The model under review builds one solid part; all positions refer to its coordinate system, in mm. A direction names the side the tool comes from. Round coordinates to 2 decimals unless told otherwise and drop trailing zeros. Order: outer loops, then holes, each group sorted by start corner. A loop starts at its lowest first (then second) coordinate and runs counter-clockwise, first axis right, second up. Notation, with made-up numbers: (60, -35) -> (109, -35) arc R23 ccw to (109, -22) -> close; hole circle Ø8 at (-17, 61.5). An arc over 180 degrees is marked (long way). Use a Markdown table: item, result. Add a question column.
```python
from build123d import *

# Parameters (mm, degrees)
F1_DEPTH = 25.4
F2_DEPTH = 25.4


with BuildPart() as f1:
    # F0 (on Front) → F1 (new body)
    with BuildSketch(Plane.XZ):
        Polygon((-174.676194787, -63.6054873466), (-136.6764605045, -58.7648972869), (-154.4505208731, -22.218702361), (-142.8054571152, 37.529643625), (-136.6764605045, 37.9512919024), (-124.7218182419, 38.7737192321), (60.676984489, 51.5283495188), (90.0961384177, 81.2006369233), (-136.6764605045, 63.0854219198), (-164.5756051188, 29.4337924282), align=None)
        Polygon((-124.7218182419, 38.7737192321), (-136.6764605045, 37.9512919024), (-66.8059885502, -58.7648972869), (-56.2220695239, -45.9986950765), align=None)
        Polygon((90.0961384177, 63.0854219198), (90.0961384177, 81.2006369233), (60.676984489, 51.5283495188), (62.1969938034, 29.4337924282), align=None)
    extrude(amount=F1_DEPTH)

    # F2 (add): a face of the model
    f2_faces = [f1.faces().sort_by_distance(p)[0] for p in [
        (-166.6256944507, -25.4, -17.4115576837),
    ]]
    extrude(f2_faces, amount=F2_DEPTH)


solid = f1.part
```
Q1. Wall thickness on line 1 (X direction, y = -38, z = -10); line 2 (Z direction, x = -74, y = -15.5); line 3 (X direction, y = -17.5, z = -11.5): over which ranges is each line inside the solid? List them lowest first. Write a range as [from, to].
Q2. Add section D-D (x = 11.5). Write out the cut boundary in (y, z), then the cut area to 3 significant figures.
Q3. Add section A-A (x = -146). Write out the cut boundary in (y, z).
Q4. Mouldability with a two-part tool opening along Z and no side actions: class faces 1 (the flat face through (-61.588, -25.044, -52.471)), 2 (the flat face through (90.096, -25, 72)), 3 (the flat face through (-148.71, -25.04, 7.24)) as pulls with the +Z half, pulls with the -Z half, needs draft (parallel to the pull), parting line crosses it, or undercut.
Q5. Add section C-C (z = 47). Write out the cut boundary in (x, y).
Q6. Add section B-B (y = -15.5). Write out the cut boundary in (x, z), then the cut area to 3 significant figures.
Q7. Insertion check: pin 1 (10 mm diameter, centred on x = -0.5, y = -44, fed in from -Z); pin 2 (1 mm diameter, centred on y = -12, z = -4.5, fed in from -X); pin 3 (1.5 mm diameter, centred on x = 10.5, y = -34, fed in from +Z). Each pin has a flat end and moves straight along its axis. Give the tip position at first contact, or say it passes through.
Q8. Machinability: for faces 4 (the flat face through (75.95, -25.04, 46.02)), 5 (the flat face through (61.426, -25.044, 40.636)), 6 (the flat face through (-139.784, -25.044, 37.738)), which of the approach directions +Z, -Z, +X, -X, +Y, -Y give a long, thin tool a straight path to every point of the face, cutting with its end or side? Answer none if there is none.
Report:
| question | item | result |
|---|---|---|
| 1 | line 1 | x = [-168.86, -152.07], [-102.04, -85.31] |
| 1 | line 2 | z = [-48.81, -24], [42.26, 68.09] |
| 1 | line 3 | x = [-169.02, -152.36], [-100.95, -84.1] |
| 2 | outline | (-50.8, 48.15) -> (0, 48.15) -> (0, 74.92) -> (-50.8, 74.92) -> close |
| 2 | area | 1,360 mm² |
| 3 | outline | (-50.8, -59.95) -> (0, -59.95) -> (0, -39.59) -> (-50.8, -39.59) -> close; (-50.8, 21.14) -> (0, 21.14) -> (0, 51.84) -> (-50.8, 51.84) -> close |
| 4 | face 1 | pulls with the -Z half |
| 4 | face 2 | needs draft |
| 4 | face 3 | undercut |
| 5 | outline | (-150.01, -50.8) -> (-5.15, -50.8) -> (-5.15, 0) -> (-150.01, 0) -> close; (60.99, -50.8) -> (76.76, -50.8) -> (76.76, 0) -> (60.99, 0) -> close |
| 6 | outline | (-174.68, -63.61) -> (-136.68, -58.76) -> (-154.45, -22.22) -> (-142.81, 37.53) -> (-136.68, 37.95) -> (-66.81, -58.76) -> (-56.22, -46) -> (-124.72, 38.77) -> (60.68, 51.53) -> (62.2, 29.43) -> (90.1, 63.09) -> (90.1, 81.2) -> (-136.68, 63.09) -> (-164.58, 29.43) -> close |
| 6 | area | 10,100 mm² |
| 7 | pin 1 | stops at z = 46.98 |
| 7 | pin 2 | stops at x = -168.31 |
| 7 | pin 3 | stops at z = 74.9 |
| 8 | face 4 | -Z, +X, +Y, -Y |
| 8 | face 5 | -Z, +Y, -Y |
| 8 | face 6 | +Y, -Y |
